```python
from build123d import *

# Parameters (mm, degrees)
BOSS_EXTRUDE1_DEPTH      = 20
BOSS_EXTRUDE1_DEPTH_BACK = 20
SKETCH1_R                = 5
SKETCH1_R_2              = 6.5
CUT_EXTRUDE2_DEPTH       = 343.928564136
CUT_EXTRUDE2_DEPTH_BACK  = 343.928564136


with BuildPart() as part:
    # Sketch1 → Boss-Extrude1 (new, two sides: drawn at the far end of the back side and taken through both)
    # profile 1 of 5: a face of its own
    with BuildSketch(Plane(origin=(0, 0, 0), x_dir=(1, 0, 0), z_dir=(0, 1, 0)).offset(-BOSS_EXTRUDE1_DEPTH_BACK)):
        with BuildLine():
            add(Edge.make_bspline(
                [(-328.284271247, 28.284271247), (-322.910070204, 33.658472291), (-311.873452078, 37.427029787), (-296.732235412, 39.86629798)],
                knots=[0, 0, 0, 0, 0.1900067, 0.1900067, 0.1900067, 0.1900067], degree=3))
            ThreePointArc((-328.284271247, 28.284271247), (-328.284271247, -28.284271247), (-271.715728753, -28.284271247))
            ThreePointArc((-271.715728753, -28.284271247), (-263.0448187, -15.307337295), (-260, 0))
            ThreePointArc((-260, 0), (-270.583078139, 27.104330064), (-296.732235412, 39.86629798))
        make_face()
    # profile 2 of 5: a face of its own
    with BuildSketch(Plane(origin=(0, 0, 0), x_dir=(1, 0, 0), z_dir=(0, 1, 0)).offset(-BOSS_EXTRUDE1_DEPTH_BACK)):
        with BuildLine():
            ThreePointArc((-260, 0), (-263.0448187, -15.307337295), (-271.715728753, -28.284271247))
            add(Edge.make_bspline(
                [(-271.715728753, -28.284271247), (-194.91847241, 48.512985095), (-42.964488834, -10.495172733), (-6.202879594, -19.013791961)],
                knots=[0, 0, 0, 0, 0.930923327, 0.930923327, 0.930923327, 0.930923327], degree=3))
            ThreePointArc((-6.202879594, -19.013791961), (-19.751909265, 3.140394942), (0, 20))
            add(Edge.make_bspline(
                [(-296.732235412, 39.86629798), (-232.185648118, 50.264830728), (-93.046467117, 36.506278231), (0, 20)],
                knots=[0.1900067, 0.1900067, 0.1900067, 0.1900067, 1, 1, 1, 1], degree=3))
            ThreePointArc((-296.732235412, 39.86629798), (-270.583078139, 27.104330064), (-260, 0))
        make_face()
    # profile 3 of 5: a face of its own
    with BuildSketch(Plane(origin=(0, 0, 0), x_dir=(1, 0, 0), z_dir=(0, 1, 0)).offset(-BOSS_EXTRUDE1_DEPTH_BACK)):
        with BuildLine():
            ThreePointArc((0, 20), (-19.751909265, 3.140394942), (-6.202879594, -19.013791961))
            add(Edge.make_bspline(
                [(-6.202879594, -19.013791961), (-3.475082803, -19.645893294), (-1.381533462, -20), (0, -20)],
                knots=[0.930923327, 0.930923327, 0.930923327, 0.930923327, 1, 1, 1, 1], degree=3))
            add(Edge.make_bspline(
                [(0, -20), (0.844585297, -20), (2.387633143, -19.856968751)],
                knots=[0, 0, 0, 0.142944169, 0.142944169, 0.142944169], degree=2))
            ThreePointArc((2.387633143, -19.856968751), (14.9624975, -13.271159278), (20, 0))
            ThreePointArc((20, 0), (16.104446086, 11.859461044), (5.935318374, 19.0990051))
            add(Edge.make_bspline(
                [(0, 20), (0.011302239, 20), (5.935318374, 19.0990051)],
                knots=[0, 0, 0, 0.358766717, 0.358766717, 0.358766717], degree=2))
        make_face()
        with Locations(Location((0, 0, 0), (0, 0, 270))):
            Circle(SKETCH1_R, mode=Mode.SUBTRACT)
    # profile 4 of 5: a face of its own
    with BuildSketch(Plane(origin=(0, 0, 0), x_dir=(1, 0, 0), z_dir=(0, 1, 0)).offset(-BOSS_EXTRUDE1_DEPTH_BACK)):
        with BuildLine():
            add(Edge.make_bspline(
                [(5.935318374, 19.0990051), (16.523469771, 17.488632981), (46, 13)],
                knots=[0.358766717, 0.358766717, 0.358766717, 1, 1, 1], degree=2))
            ThreePointArc((5.935318374, 19.0990051), (16.104446086, 11.859461044), (20, 0))
            ThreePointArc((20, 0), (14.9624975, -13.271159278), (2.387633143, -19.856968751))
            add(Edge.make_bspline(
                [(2.387633143, -19.856968751), (11.639344201, -18.999390814), (46, -13)],
                knots=[0.142944169, 0.142944169, 0.142944169, 1, 1, 1], degree=2))
            ThreePointArc((46, -13), (33, 0), (46, 13))
        make_face()
    # profile 5 of 5: a face of its own
    with BuildSketch(Plane(origin=(0, 0, 0), x_dir=(1, 0, 0), z_dir=(0, 1, 0)).offset(-BOSS_EXTRUDE1_DEPTH_BACK)):
        with BuildLine():
            ThreePointArc((59, 0), (55.192388155, 9.192388155), (46, 13))
            ThreePointArc((46, 13), (33, 0), (46, -13))
            ThreePointArc((46, -13), (55.192388155, -9.192388155), (59, 0))
        make_face()
        with Locations(Location((46, 0, 0), (0, 0, 270))):
            Circle(SKETCH1_R_2, mode=Mode.SUBTRACT)
    extrude(amount=BOSS_EXTRUDE1_DEPTH + BOSS_EXTRUDE1_DEPTH_BACK)

    # Sketch3 → Cut-Extrude2 (cut, two sides: drawn at the far end of the back side and taken through both)
    with BuildSketch(Plane(origin=(-71.299423149, 0, -172.132034356), x_dir=(0.7071067811865464, 0, -0.7071067811865488), z_dir=(0.7071067811865488, 0, 0.7071067811865464)).offset(-CUT_EXTRUDE2_DEPTH_BACK)):
        with BuildLine():
            add(Edge.make_bspline(
                [(-283.431457505, -20), (-227.543374676, -10.63873359), (-151.71769793, -12.794597658), (-85.441558773, -20)],
                knots=[0, 0, 0, 0, 1, 1, 1, 1], degree=3))
            Line((-85.441558773, -20), (-283.431457505, -20))
        make_face()
        with BuildLine():
            Line((-283.431457505, 20), (-85.441558773, 20))
            add(Edge.make_bspline(
                [(-283.431457505, 20), (-227.543374676, 10.63873359), (-151.71769793, 12.794597658), (-85.441558773, 20)],
                knots=[0, 0, 0, 0, 1, 1, 1, 1], degree=3))
        make_face()
    extrude(amount=CUT_EXTRUDE2_DEPTH + CUT_EXTRUDE2_DEPTH_BACK, mode=Mode.SUBTRACT)


solid = part.part
```
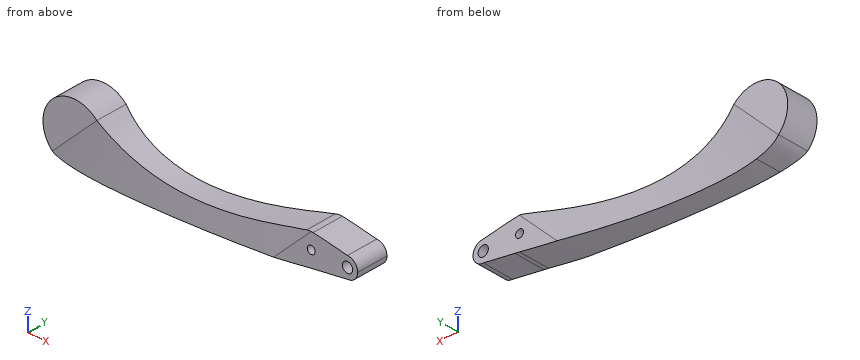
Could you check a few things on this model? Use its own coordinates, in mm. Round coordinates to 2 decimals unless told otherwise and drop trailing zeros. Answer in a Markdown table with one row per item. Add a question column.
Q1. Will these pins go through, and if not, where does the flat tip stop? pin 1 Ø1.5 at (x, z) = (-220, -26) entering from -Y; pin 2 Ø9 at (x, z) = (0, 0) entering from +Y; pin 3 Ø10 at (x, z) = (-257, -6.5) entering from +Y; pin 4 Ø8 at (x, y) = (-295.5, -8) entering from +Z.
Q2. If I drill on line 1 (Y direction, x = -207, z = -19); line 2 (X direction, y = -3, z = 28); line 3 (X direction, y = -15.5, z = 33.5), over which ranges is the centre line in solid material (lowest first)? Write a range as from..to.
Q3. Imagine slicing it at A-A (y = 2). Give the number of separate pieces and of enclosed holes in the cut face, then the cut area to 3 significant figures.
Values:
| question | item | result |
|---|---|---|
| 1 | pin 1 | y = -13.89 |
| 1 | pin 2 | through |
| 1 | pin 3 | y = 16.2 |
| 1 | pin 4 | z = 40 |
| 2 | line 1 | -13.82..13.82 |
| 2 | line 2 | -328.57..-271.43 |
| 2 | line 3 | -321.86..-278.14 |
| 3 | separate pieces | 1 |
| 3 | enclosed holes | 2 |
| 3 | area | 16,300 mm^2 |
